Here's how the part is built. I have some questions about the finished solid (model axes, mm). Face numbers are marked on the shaded views. A direction names the side the tool comes from. Give positions to 0.01 mm unless a question says otherwise; leave off trailing zeros. Loops run counter-clockwise (first coordinate to the right, second up) from the corner with the lowest first, then second, coordinate; pieces in that order, holes last. Notation, with made-up numbers: (14.25, -35.5) -> (56.25, -35.5) arc R26 cw to (56.25, 1.5) -> close; hole circle Ø8 at (-29, -17.75). An arc over 180 degrees is marked (long way). Answer in a Markdown table with one row per item. Add a question column.
Item 1: If we section it at B-B (z = 5.75): Write out the boundary of the cut face in (x, y).
Item 2: We'd pull the mould along X, two halves only. Please class the marked faces 1, 2, 3 and 4: released by +X, released by -X, zero draft, split by the parting line, or undercut.
Item 3: If I drill on line 1 (X direction, y = -5.75, z = -3); line 2 (X direction, y = -6.25, z = 7); line 3 (X direction, y = -5, z = 8.75), over which ranges is the centre line in solid material (lowest first)?
Item 4: If we section it at C-C (x = 0.75): Write out the boundary of the cut face in (y, z), then the cut area to 3 significant figures.
Item 5: If we section it at D-D (y = -1.5): Write out the boundary of the cut face in (x, z), then the cut area to 3 significant figures.
Item 6: Which directions (+Z, -Z, +X, -X, +Y, -Y) give clear straight access to the entire face, cutting with the end or side of a thin tool? Please do the marked faces 5, 6, 7, 8 and 9.
Item 7: If we section it at A-A (y = -6.25): Write out the boundary of the cut face in (x, z) (3 decimals).
Item 8: For P1, Ø0.5, axis at x = -0.5, z = -0.5, coming from the -Y side; P2, Ø2, axis at x = 8, z = 12, coming from the +Y side; P3, Ø3, axis at x = -4.5, y = -4.5, coming from the -Z side, each with a flat end and sliding along its axis, tell me the tip position at first contact or that it passes through.
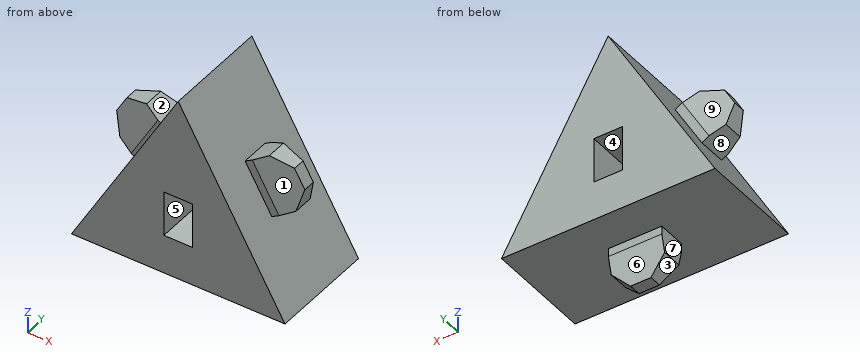
```python
from build123d import *

# Parameters (mm, degrees)
F1_DEPTH    = 13
F2_W        = 3.5
F2_H        = 5.5
F3_DEPTH    = 13.001
F4_W        = 3.5
F4_H        = 6.5
F6_DEPTH    = 5
F5_W        = 3.5
F5_H        = 6.5
F7_DEPTH    = 5
F8_W        = 6.5
F8_H        = 3.5
F9_DEPTH    = 5
F10_SIZE2   = 1
F10_SIZE    = 4
F10_2_SIZE2 = 1
F10_2_SIZE  = 4
F10_3_SIZE2 = 1
F10_3_SIZE  = 4
F10_4_SIZE2 = 1
F10_4_SIZE  = 4
F11_SIZE2   = 4
F11_SIZE    = 1
F11_2_SIZE2 = 4
F11_2_SIZE  = 1
F12_SIZE    = 2


with BuildPart() as f1:
    # F0 (on Front) → F1 (new body)
    with BuildSketch(Plane.XZ):
        Polygon((0, 7.5055534995), (0, 22.5166604984), (-13, 0), align=None)
        Polygon((13, 0), (0, 22.5166604984), (0, 7.5055534995), align=None)
        Polygon((0, 7.5055534995), (-13, 0), (13, 0), align=None)
    extrude(amount=F1_DEPTH)

    # F2 (on face) → F3 (cut, through all)
    with BuildSketch(Plane.XZ.offset(13)):
        with Locations((0, 7.5106434524)):
            Rectangle(F2_W, F2_H)
    extrude(amount=-F3_DEPTH, mode=Mode.SUBTRACT)

    # F4 (on face) → F6 (join)
    with BuildSketch(Plane(origin=(9.75, 0, 5.6291651246), x_dir=(0, 1, 0), z_dir=(0.8660254038, 0, 0.5))):
        with Locations((-6.5, 6.5)):
            Rectangle(F4_W, F4_H)
    extrude(amount=F6_DEPTH)

    # F5 (on face) → F7 (join)
    with BuildSketch(Plane(origin=(-9.75, 0, 5.6291651246), x_dir=(0, -1, 0), z_dir=(-0.8660254038, 0, 0.5))):
        with Locations((6.5, 6.5)):
            Rectangle(F5_W, F5_H)
    extrude(amount=F7_DEPTH)

    # F8 (on face) → F9 (join)
    with BuildSketch(Plane(origin=(0, 0, 0), x_dir=(1, 0, 0), z_dir=(0, 0, -1))):
        with Locations((0, 6.5)):
            Rectangle(F8_W, F8_H)
    extrude(amount=F9_DEPTH)

    # F10
    f10_edges = [f1.edges().sort_by_distance(p)[0] for p in [
        (10.830127, -8.25, 13.75833),
    ]]
    f10_side = f1.faces().sort_by_distance((8.665064, -8.25, 12.50833))[0]
    chamfer(f10_edges, length=F10_SIZE, length2=F10_SIZE2, reference=f10_side)

    # F10#2
    f10_2_edges = [f1.edges().sort_by_distance(p)[0] for p in [
        (10.830127, -4.75, 13.75833),
    ]]
    f10_2_side = f1.faces().sort_by_distance((8.665064, -4.75, 12.50833))[0]
    chamfer(f10_2_edges, length=F10_2_SIZE, length2=F10_2_SIZE2, reference=f10_2_side)

    # F10#3
    f10_3_edges = [f1.edges().sort_by_distance(p)[0] for p in [
        (0, -4.75, -5),
    ]]
    f10_3_side = f1.faces().sort_by_distance((0, -4.75, -2.5))[0]
    chamfer(f10_3_edges, length=F10_3_SIZE, length2=F10_3_SIZE2, reference=f10_3_side)

    # F10#4
    f10_4_edges = [f1.edges().sort_by_distance(p)[0] for p in [
        (-10.830127, -4.75, 13.75833),
    ]]
    f10_4_side = f1.faces().sort_by_distance((-8.665064, -4.75, 12.50833))[0]
    chamfer(f10_4_edges, length=F10_4_SIZE, length2=F10_4_SIZE2, reference=f10_4_side)

    # F11
    f11_edges = [f1.edges().sort_by_distance(p)[0] for p in [
        (-10.830127, -8.25, 13.75833),
    ]]
    f11_side = f1.faces().sort_by_distance((-10.830127, -7, 13.75833))[0]
    chamfer(f11_edges, length=F11_SIZE, length2=F11_SIZE2, reference=f11_side)

    # F11#2
    f11_2_edges = [f1.edges().sort_by_distance(p)[0] for p in [
        (0, -8.25, -5),
    ]]
    f11_2_side = f1.faces().sort_by_distance((0, -7, -5))[0]
    chamfer(f11_2_edges, length=F11_2_SIZE, length2=F11_2_SIZE2, reference=f11_2_side)

    # F12
    f12_edges = [f1.edges().sort_by_distance(p)[0] for p in [
        (-9.205127, -6.5, 16.572913),
        (-12.455127, -6.5, 10.943748),
        (9.205127, -6.5, 16.572913),
        (12.455127, -6.5, 10.943748),
        (-3.25, -6.5, -5),
        (3.25, -6.5, -5),
    ]]
    chamfer(f12_edges, length=F12_SIZE)


solid = f1.part
```
Recorded:
| question | item | result |
|---|---|---|
| 1 | outline | (-9.68, -13) -> (-1.75, -13) -> (-1.75, 0) -> (-9.68, 0) -> close; (1.75, -13) -> (9.68, -13) -> (9.68, 0) -> (1.75, 0) -> close |
| 2 | face 1 | released by +X |
| 2 | face 2 | undercut |
| 2 | face 3 | released by -X |
| 2 | face 4 | undercut |
| 3 | line 1 | x = -3.25 to 3.25 |
| 3 | line 2 | x = -8.96 to -1.75, 1.75 to 8.96 |
| 3 | line 3 | x = -8.66 to -1.75, 1.75 to 8.66 |
| 4 | outline | (-13, 0) -> (-8.25, 0) -> (-8.25, -1) -> (-7.25, -5) -> (-5.75, -5) -> (-4.75, -1) -> (-4.75, 0) -> (0, 0) -> (0, 4.76) -> (-13, 4.76) -> close; (-13, 10.26) -> (0, 10.26) -> (0, 21.22) -> (-13, 21.22) -> close |
| 4 | area | 218 mm^2 |
| 5 | outline | (-13, 0) -> (13, 0) -> (0, 22.52) -> close; hole (-1.75, 4.76) -> (1.75, 4.76) -> (1.75, 10.26) -> (-1.75, 10.26) -> close |
| 5 | area | 273 mm^2 |
| 6 | face 5 | +Y, -Y |
| 6 | face 6 | -Z, +X, -X, +Y |
| 6 | face 7 | -Z, -X, +Y, -Y |
| 6 | face 8 | -X, +Y, -Y |
| 6 | face 9 | +Z, -X, +Y |
| 7 | outline | (-13, 0) -> (-3.25, 0) -> (-3.25, -3) -> (-1.25, -5) -> (1.25, -5) -> (3.25, -3) -> (3.25, 0) -> (13, 0) -> (8.125, 8.444) -> (10.723, 9.944) -> (11.455, 12.676) -> (10.205, 14.841) -> (7.473, 15.573) -> (4.875, 14.073) -> (0, 22.517) -> (-4.875, 14.073) -> (-7.473, 15.573) -> (-10.205, 14.841) -> (-11.455, 12.676) -> (-10.723, 9.944) -> (-8.125, 8.444) -> close; hole (-1.75, 4.761) -> (1.75, 4.761) -> (1.75, 10.261) -> (-1.75, 10.261) -> close |
| 8 | P1 | stops at y = -8.25 |
| 8 | P2 | stops at y = -4.75 |
| 8 | P3 | stops at z = -3.04 |
